Autodesk Inventor part; units mm, degrees
ref_plane "EbeneAuflage" through (-20, -13, 0) normal (0, 0, 1) x (1, 0, 0)
ref_plane "YZ Plane" through (0, 0, 0) normal (1, 0, 0) x (0, 1, 0)
ref_plane "XZ Plane" through (0, 0, 0) normal (0, 1, 0) x (-1, 0, 0)
ref_plane "EbeneBoden" through (-11.5031, -4.6031, 1.9) normal (0, 0, 1) x (1, 0, 0)
ref_plane "EbeneWändeEnde" through (17.7, 4.9, -6.9) normal (0, 0, -1) x (-1, 0, 0)
sketch "SkizzeBoden" plane through (-11.5031, -4.6031, 1.9) normal (0, 0, 1) x (1, 0, 0)
  line L0 (-7.1969, 7.4031) -> (6.8031, 7.4031)
  line L1 (6.8031, 7.4031) -> (6.8031, -7.7969)
  line L2 (6.8031, -7.7969) -> (4.3031, -7.7969)
  line L3 (4.3031, -7.7969) -> (4.3031, -6.7969)
  line L4 (4.3031, -6.7969) -> (-7.1969, -6.7969)
  line L5 (-7.1969, -6.7969) -> (-7.1969, 7.4031)
  line L6 (31.5031, 17.6031) -> (-8.4969, 17.6031)
  line L7 (-8.4969, 17.6031) -> (-8.4969, -8.3969)
  line L8 (-8.4969, -8.3969) -> (31.5031, -8.3969)
  line L9 (31.5031, -8.3969) -> (31.5031, 17.6031)
  line L10 (-18.7369, 4.6031) -> (41.7431, 4.6031)
  line L11 (11.5031, -15.8369) -> (11.5031, 25.0431)
  line L12 (-10.0969, 19.2031) -> (33.1031, 19.2031)
  line L13 (33.1031, 19.2031) -> (33.1031, -9.9969)
  line L14 (33.1031, -9.9969) -> (-10.0969, -9.9969)
  line L15 (-10.0969, -9.9969) -> (-10.0969, 19.2031)
  point P0 (11.5031, 4.6031)
  dimension "d0" = 1.6
extrude "Boden" add sketch "SkizzeBoden" along normal blind 1.5
sketch "SkizzeWände" plane through (-11.5031, -4.6031, 1.9) normal (0, 0, -1) x (-1, 0, 0)
  line L0 (10.0969, 19.2031) -> (-33.1031, 19.2031)
  line L1 (-33.1031, 19.2031) -> (-33.1031, -9.9969)
  line L2 (-33.1031, -9.9969) -> (10.0969, -9.9969)
  line L3 (10.0969, -9.9969) -> (10.0969, 19.2031)
  line L4 (-31.6031, 17.7031) -> (8.5969, 17.7031)
  line L5 (8.5969, 17.7031) -> (8.5969, -8.4969)
  line L6 (8.5969, -8.4969) -> (-31.6031, -8.4969)
  line L7 (-31.6031, -8.4969) -> (-31.6031, 17.7031)
  point P0 (-11.5031, 4.6031)
  dimension "d3" = 1.5
extrude "Wände" add sketch "SkizzeWände" along normal up to surface (8.8 mm away)
sketch "SkizzeAuflage" plane through (-11.5031, -4.6031, 1.9) normal (0, 0, -1) x (-1, 0, 0)
  line L0 (8.5969, -8.4969) -> (8.5969, 17.7031)
  line L1 (-31.6031, -8.4969) -> (8.5969, -8.4969)
  line L2 (-31.6031, 17.7031) -> (-31.6031, -8.4969)
  line L3 (8.5969, 17.7031) -> (-31.6031, 17.7031)
  line L4 (10.0969, 19.2031) -> (10.0969, -9.9969)
  line L5 (-33.1031, 19.2031) -> (10.0969, 19.2031)
  line L6 (-33.1031, -9.9969) -> (-33.1031, 19.2031)
  line L7 (10.0969, -9.9969) -> (-33.1031, -9.9969)
  line L8 (-26.6031, 3.5031) -> (-25.1031, 3.5031)
  line L9 (-25.1031, 3.5031) -> (-25.1031, -6.4969)
  line L10 (-25.1031, -6.4969) -> (-26.6031, -6.4969)
  line L11 (-26.6031, -6.4969) -> (-26.6031, 3.5031)
  line L12 (-17.1031, 3.5031) -> (-15.6031, 3.5031)
  line L13 (-15.6031, 3.5031) -> (-15.6031, -6.4969)
  line L14 (-15.6031, -6.4969) -> (-17.1031, -6.4969)
  line L15 (-17.1031, -6.4969) -> (-17.1031, 3.5031)
  line L16 (6.5969, 13.7031) -> (-13.4031, 13.7031)
  line L17 (-13.4031, 13.7031) -> (-13.4031, 12.2031)
  line L18 (-13.4031, 12.2031) -> (6.5969, 12.2031)
  line L19 (6.5969, 12.2031) -> (6.5969, 13.7031)
  point P0 (-11.5031, 4.6031)
  dimension "d6" = 5
  dimension "d7" = 1.5
  dimension "d8" = 8
  dimension "d9" = 2
  dimension "d10" = 10
  dimension "d11" = 20
  dimension "d12" = 1.5
  dimension "d13" = 4
  dimension "d14" = 2
ref_plane "EbeneAuflage" through (-20, -13, 0) normal (0, 0, 1) x (1, 0, 0)
extrude "Auflage" add sketch "SkizzeAuflage" along normal up to surface (1.9 mm away) contours L8 L9 L10 L11 | L12 L13 L14 L15 | L19 L18 L17 L16
sketch "SkizzeSD" plane through (-21.6, -14.6, 3.4) normal (0, -1, 0) x (1, 0, 0)
  line L0 (43.2, 0) -> (43.2, -10.3)
  line L1 (3.1, -2.6) -> (14.2, -2.6)
  line L2 (14.2, -2.6) -> (14.2, -1.6)
  line L3 (14.2, -1.6) -> (3.1, -1.6)
  line L4 (3.1, -1.6) -> (3.1, -2.6)
  line L5 (41.7, -1.5) -> (1.5, -1.5)
  line L6 (14.5, -1.5) -> (2.8, -1.5)
  line L7 (2.8, -1.5) -> (2.8, -2.9)
  line L8 (2.8, -2.9) -> (14.5, -2.9)
  line L9 (14.5, -2.9) -> (14.5, -1.5)
  line L10 (8.65, -4) -> (8.65, -0.8838) construction
  point P0 (21.6, -3.4)
  point P1 (8.65, -2.6)
  dimension "d17" = 0.3
  dimension "d18" = 0.3
extrude "SD" cut sketch "SkizzeSD" against normal up to surface (1.5 mm away) contours L4 L3 L2 L1 | L9 L8 L7 L5
sketch "Skizze7" plane through (-21.6, -14.6, 3.4) normal (0, -1, 0) x (1, 0, 0)
  line L0 (14.5, -1.5) -> (14.5, -2.9)
  line L1 (14.5, -2.9) -> (2.8, -2.9)
  line L2 (0, 0) -> (43.2, 0)
  line L3 (15.5, -3.9) -> (1.8, -3.9)
  line L4 (1.8, -3.9) -> (1.8, 0)
  line L5 (1.8, 0) -> (15.5, 0)
  line L6 (15.5, 0) -> (15.5, -3.9)
  line L7 (8.65, -3.6567) -> (8.65, -1) construction
  point P0 (21.6, -3.4)
  point P1 (8.65, -2.9)
  dimension "d21" = 1
  dimension "d22" = 1
extrude "SDHilfe" cut sketch "Skizze7" against normal blind 0.8
sketch "SkizzeLED" plane through (-21.6, -14.6, -6.9) normal (0, -1, 0) x (1, 0, 0)
  line L0 (16.6, 5.2) -> (17.6, 5.2)
  line L1 (16.6, 5.2) -> (16.6, 4.1)
  line L2 (17.6, 4.1) -> (16.6, 4.1)
  line L3 (17.6, 5.2) -> (17.6, 4.1)
  line L4 (15.1, 5.2) -> (16.1, 5.2)
  line L5 (15.1, 5.2) -> (15.1, 4.1)
  line L6 (16.1, 4.1) -> (15.1, 4.1)
  line L7 (16.1, 5.2) -> (16.1, 4.1)
  line L8 (13.6, 5.2) -> (14.6, 5.2)
  line L9 (13.6, 5.2) -> (13.6, 4.1)
  line L10 (14.6, 4.1) -> (13.6, 4.1)
  line L11 (14.6, 5.2) -> (14.6, 4.1)
  line L12 (15.6, 3.5363) -> (15.6, 5.4531) construction
  line L13 (17.7, 4.1) -> (13.5, 4.1)
  line L14 (13.5, 4.1) -> (13.5, 5.2)
  line L15 (13.5, 5.2) -> (17.7, 5.2)
  line L16 (17.7, 5.2) -> (17.7, 4.1)
  line L17 (41.6, 5.2) -> (1.6, 5.2)
  point P0 (21.6, 6.9)
  point P1 (15.6, 4.1)
  dimension "d25" = 0.1
extrude "LED" cut sketch "SkizzeLED" against normal up to surface (1.5 mm away)
fillet "RundungLED" radius 0.3 4 edges at (-8.1, -13.85, -2.8) (-3.9, -13.85, -2.8) (-8.1, -13.85, -1.7) (-3.9, -13.85, -1.7)
sketch "SkizzeUSB" plane through (-21.6, 14.6, 3.4) normal (0, 1, 0) x (1, 0, 0)
  line L0 (43.2, 10.3) -> (0, 10.3)
  ellipse E0 centre (28.273, 7.641) end of major axis (28.5965, 8.1263) minor radius 0.5 (28.8, 7.72) -> (28.3475, 8.2) ccw
  line L1 (28.3475, 8.2) -> (21.3525, 8.2)
  ellipse E1 centre (21.427, 7.641) end of major axis (21.1035, 8.1263) minor radius 0.5 (21.3525, 8.2) -> (20.9, 7.72) ccw
  line L2 (20.9, 7.72) -> (20.9, 6.4602)
  line L3 (22.4652, 4.8) -> (20.9, 6.4602)
  line L4 (22.4652, 4.8) -> (27.2348, 4.8)
  line L5 (28.8, 6.4602) -> (27.2348, 4.8)
  line L6 (28.8, 6.4602) -> (28.8, 7.72)
  ellipse E2 centre (28.273, 7.641) end of major axis (28.5965, 8.1263) minor radius 0.5 (28.8, 7.72) -> (28.3475, 8.2) ccw
  line L7 (28.3475, 8.2) -> (21.3525, 8.2)
  ellipse E3 centre (21.427, 7.641) end of major axis (21.1035, 8.1263) minor radius 0.5 (21.3525, 8.2) -> (20.9, 7.72) ccw
  line L8 (20.9, 7.72) -> (20.9, 6.4602)
  line L9 (22.4652, 4.8) -> (20.9, 6.4602)
  line L10 (22.4652, 4.8) -> (27.2348, 4.8)
  line L11 (28.8, 6.4602) -> (27.2348, 4.8)
  line L12 (28.8, 6.4602) -> (28.8, 7.72)
  line L13 (20.6, 10.3) -> (29.1, 10.3)
  line L14 (29.1, 10.3) -> (29.1, 4.5)
  line L15 (29.1, 4.5) -> (20.6, 4.5)
  line L16 (20.6, 4.5) -> (20.6, 10.3)
  line L17 (24.85, 8.6856) -> (24.85, 4.4469) construction
  point P0 (21.6, 3.4)
  point P1 (24.85, 8.2)
  dimension "d29" = 0.3
  dimension "d30" = 0.3
extrude "USB" cut sketch "SkizzeUSB" against normal up to surface (1.5 mm away) contours L14 L15 L16 L0 | L6 L5 L4 L3 L2 E1 L1 E0
chamfer "FaseUSB" distance 1.5 angle 45 2 edges at (7.5, 13.85, -1.1) (-1, 13.85, -1.1)
sketch "Skizze10" plane through (-21.6, -14.6, 3.4) normal (-1, 0, 0) x (0, 0, 1)
  line L0 (-10.3, 29.2) -> (-10.3, 0)
  line L1 (-5.1, 27) -> (-5.1, 12)
  line L2 (-5.1, 27) -> (-8.8, 27)
  line L3 (-8.8, 12) -> (-8.8, 27)
  line L4 (-5.1, 12) -> (-8.8, 12)
  line L5 (-5.1, 11.2) -> (-5.1, 2.2)
  line L6 (-5.1, 11.2) -> (-8.8, 11.2)
  line L7 (-8.8, 2.2) -> (-8.8, 11.2)
  line L8 (-5.1, 2.2) -> (-8.8, 2.2)
  line L9 (-4.8, 1.9) -> (-10.3, 1.9)
  line L10 (-10.3, 1.9) -> (-10.3, 27.3)
  line L11 (-10.3, 27.3) -> (-4.8, 27.3)
  line L12 (-4.8, 27.3) -> (-4.8, 1.9)
  line L13 (0, 29.2) -> (0, 0)
  line L14 (-10.3, 29.2) -> (0, 29.2)
  line L15 (3, 14.6) -> (-13.529, 14.6) construction
  line L16 (-8.4, 2.6) -> (-8.4, 10.8)
  line L17 (-8.4, 10.8) -> (-5.5, 10.8)
  line L18 (-5.5, 10.8) -> (-5.5, 2.6)
  line L19 (-5.5, 2.6) -> (-8.4, 2.6)
  line L20 (-8.4, 12.4) -> (-8.4, 26.6)
  line L21 (-8.4, 26.6) -> (-5.5, 26.6)
  line L22 (-5.5, 26.6) -> (-5.5, 12.4)
  line L23 (-5.5, 12.4) -> (-8.4, 12.4)
  point P0 (-3.4, 14.6)
  point P1 (0, 14.6)
  dimension "d36" = 0.3
  dimension "d38" = 0.3
extrude "JSTFC" cut sketch "Skizze10" against normal up to surface (1.5 mm away) contours L11 L12 L9 L0 | L1 L4 L3 L2 | L5 L8 L7 L6 | L16 L17 L18 L19 | L20 L21 L22 L23
sketch "Skizze11" plane through (21.6, -14.6, 3.4) normal (1, 0, 0) x (0, 0, -1)
  line L0 (10.3, 0) -> (10.3, 29.2)
  line L1 (13.0125, 14.6) -> (-3.6442, 14.6) construction
  line L2 (5.1, 15) -> (5.1, 24)
  line L3 (5.1, 15) -> (8.8, 15)
  line L4 (8.8, 24) -> (8.8, 15)
  line L5 (5.1, 24) -> (8.8, 24)
  line L6 (5.1, 5.2) -> (5.1, 14.2)
  line L7 (5.1, 5.2) -> (8.8, 5.2)
  line L8 (8.8, 14.2) -> (8.8, 5.2)
  line L9 (5.1, 14.2) -> (8.8, 14.2)
  line L10 (10.3, 24.3) -> (4.8, 24.3)
  line L11 (4.8, 24.3) -> (4.8, 4.9)
  line L12 (4.8, 4.9) -> (10.3, 4.9)
  line L13 (10.3, 4.9) -> (10.3, 24.3)
  line L14 (5.5, 13.8) -> (8.4, 13.8)
  line L15 (8.4, 13.8) -> (8.4, 5.6)
  line L16 (8.4, 5.6) -> (5.5, 5.6)
  line L17 (5.5, 5.6) -> (5.5, 13.8)
  line L18 (8.4, 23.6) -> (8.4, 15.4)
  line L19 (8.4, 15.4) -> (5.5, 15.4)
  line L20 (5.5, 15.4) -> (5.5, 23.6)
  line L21 (5.5, 23.6) -> (8.4, 23.6)
  point P0 (3.4, 14.6)
  point P1 (10.3, 14.6)
  dimension "d41" = 0.3
  dimension "d42" = 0.3
extrude "JSTOSD" cut sketch "Skizze11" against normal up to surface (1.5 mm away) contours L12 L11 L10 L0 | L2 L5 L4 L3 | L6 L9 L8 L7 | L14 L15 L16 L17 | L18 L19 L20 L21
sketch "Skizze12" plane through (21.6, -14.6, -6.9) normal (0, 0, -1) x (-1, 0, 0)
  line L0 (0, 0) -> (0, 4.9)
  line L1 (43.2, 0) -> (0, 0)
  line L2 (21.6, -5.84) -> (21.6, 35.04)
  line L3 (51.84, 14.6) -> (-8.64, 14.6)
  line L4 (0.8, 28.4) -> (42.4, 28.4)
  line L5 (42.4, 28.4) -> (42.4, 0.8)
  line L6 (42.4, 0.8) -> (0.8, 0.8)
  line L7 (0.8, 0.8) -> (0.8, 28.4)
  point P0 (21.6, 14.6)
  dimension "d45" = 0.8
  dimension "d46" = 0.8
extrude "Lippe" cut sketch "Skizze12" against normal blind 0.6
sketch "SkizzeSchnapper" plane through (-21.6, -14.6, -6.9) normal (0, -1, 0) x (1, 0, 0)
  line L0 (36.2, 5.2) -> (41.6, 5.2)
  line L1 (36.2, 5.2) -> (36.2, 1.5)
  line L2 (42.4, 1.5) -> (36.2, 1.5)
  line L3 (42.4, 5.2) -> (42.4, 1.5)
  line L4 (41.6, 5.2) -> (42.4, 5.2)
  line L5 (0.8, 5.2) -> (1.6, 5.2)
  line L6 (0.8, 5.2) -> (0.8, 1.5)
  line L7 (7, 1.5) -> (0.8, 1.5)
  line L8 (7, 5.2) -> (7, 1.5)
  line L9 (1.6, 5.2) -> (7, 5.2)
  ellipse E0 centre (28.273, 2.659) end of major axis (28.5965, 2.1737) minor radius 0.5 (28.3475, 2.1) -> (28.8, 2.58) ccw
  line L10 (28.3475, 2.1) -> (21.3525, 2.1)
  ellipse E1 centre (21.427, 2.659) end of major axis (21.1035, 2.1737) minor radius 0.5 (20.9, 2.58) -> (21.3525, 2.1) ccw
  line L11 (20.9, 2.58) -> (20.9, 3.8398)
  line L12 (22.4652, 5.5) -> (20.9, 3.8398)
  line L13 (22.4652, 5.5) -> (27.2348, 5.5)
  line L14 (28.8, 3.8398) -> (27.2348, 5.5)
  line L15 (28.8, 3.8398) -> (28.8, 2.58)
  line L16 (35, 2.4) -> (30.5, 2.4)
  line L17 (30.5, 2.4) -> (30.5, 4)
  line L18 (30.5, 4) -> (35, 4)
  line L19 (35, 4) -> (35, 2.4)
  line L20 (21.6, -2.06) -> (21.6, 12.36)
  line L21 (1.5, 0.6) -> (0.8, 0.6)
  line L22 (41.7, 0.6) -> (1.5, 0.6)
  line L23 (42.4, 0.6) -> (41.7, 0.6)
  line L24 (0.8, 0.6) -> (42.4, 0.6)
  line L25 (41.6, 5.2) -> (1.6, 5.2)
  line L26 (8.2, 2.4) -> (12.7, 2.4)
  line L27 (12.7, 2.4) -> (12.7, 4)
  line L28 (12.7, 4) -> (8.2, 4)
  line L29 (8.2, 4) -> (8.2, 2.4)
  point P0 (21.6, 6.9)
  dimension "d49" = 4.5
  dimension "d50" = 1.8
  dimension "d51" = 1.2
  dimension "d52" = 1.6
  dimension "d53" = 1.2
extrude "Schnapper" cut sketch "SkizzeSchnapper" against normal up to surface (29.2 mm away) contours L16 L17 L18 L19 | L29 L28 L27 L26
sketch "SkizzeAufkleber" plane through (-11.5031, -4.6031, 3.4) normal (0, 0, 1) x (1, 0, 0)
  line L0 (33.1031, 19.2031) -> (-10.0969, 19.2031)
  line L1 (-10.0969, 19.2031) -> (-10.0969, -9.9969)
  line L2 (11.5031, -15.8369) -> (11.5031, 25.0431)
  line L3 (-18.7369, 4.6031) -> (41.7431, 4.6031)
  line L4 (-8.0969, 17.2031) -> (31.1031, 17.2031)
  line L5 (31.1031, 17.2031) -> (31.1031, -7.9969)
  line L6 (31.1031, -7.9969) -> (-8.0969, -7.9969)
  line L7 (-8.0969, -7.9969) -> (-8.0969, 17.2031)
  point P0 (11.5031, 4.6031)
  dimension "d56" = 2
  dimension "d57" = 2
extrude "Aufkleber" cut sketch "SkizzeAufkleber" against normal blind 0.3 contours L4 L5 L3 L2 | L2 L3 L7 L4 | L3 L5 L6 L2 | L2 L6 L7 L3
properties part number "Boden"
Work out the finished part from the listing and answer in its coordinate system (mm). A direction names the side the tool comes from. Coordinates: 2 decimals unless noted, no trailing zeros. Order: outer loops, then holes, each group sorted by start corner. A loop starts at its lowest first (then second) coordinate and runs counter-clockwise, first axis right, second up. Notation, with made-up numbers: (30, 17.25) - (35, 17.25) arc R20 ccw to (35, 42.25) - close; hole circle Ø3 at (-20.75, -37.5). An arc over 180 degrees is marked (long way). Put each result on its own line as item: value. Start each with the question number.
1) For a pull along X with two mould halves and no side action, classify faces 1 (the flat face through (-0.3, 14.6, -1.68)), 2 (the flat face through (-11, 14, -2.9)) as released by +X, released by -X, zero draft, split by the parting line, or undercut.
2) Find section A-A (x = -16.5). Give the vertices of the cut face in (y, z), plus the area to 4 significant figures.
3) Find section D-D (y = -12). Give the vertices of the cut face in (x, z), plus the area to 3 significant figures.
4) Find section B-B (z = 1.25). Give the vertices of the cut face in (x, y).
5) For faces 3 (the flat face through (-13, -13.8, 2.3)), 4 (the flat face through (11, 14, -4.5)), 5 (the flat face through (21, -9.7, -4)), 6 (the flat face through (-21, -12.7, -4)), 7 (the flat face through (-8, 9.1, 1)), determine the directions among +Z, -Z, +X, -X, +Y, -Y from which every point of the face is accessible in a straight line to the end or side of a thin tool.
6) Find the intervals of material crossed by line 1 (Y direction, x = -1.5, z = 1.5); line 2 (X direction, y = -2.75, z = 3.25); line 3 (X direction, y = 2.25, z = 0.25), in increasing order. Write a range as from..to.
7) Flat-ended cylindrical pins translate along their axes: pin 1 (5 mm diameter, centred on x = 3, y = -10, fed in from +Z); pin 2 (0.6 mm diameter, centred on x = -10.5, z = 1, fed in from -Y); pin 3 (3 mm diameter, centred on y = -10, z = -5.5, fed in from -X). Find the tip coordinate at first contact, or state that the pin passes through.
8) Find section C-C (x = 11.5). Give the vertices of the cut face in (y, z).
Results list:
1. face 1: zero draft
1. face 2: undercut
2. outline: (-14.6, -6.9) - (-13.8, -6.9) - (-13.8, -6.3) - (-13.1, -6.3) - (-13.1, 0.5) - (-13.8, 0.5) - (-13.8, -0.5) - (-14.6, -0.5) - close; (-13.8, 1.9) - (7.6, 1.9) - (7.6, 0) - (9.1, 0) - (9.1, 1.9) - (13.1, 1.9) - (13.1, -6.3) - (13.8, -6.3) - (13.8, -6.9) - (14.6, -6.9) - (14.6, 3.4) - (12.6, 3.4) - (12.6, 3.1) - (-12.6, 3.1) - (-12.6, 3.4) - (-13.8, 3.4) - close
2. area: 60.55 mm^2
3. outline: (-21.6, -1.4) - (-20.1, -1.4) - (-20.1, 1.9) - (20.1, 1.9) - (20.1, -6.3) - (20.8, -6.3) - (20.8, -6.9) - (21.6, -6.9) - (21.6, 3.4) - (19.6, 3.4) - (19.6, 3.1) - (-19.6, 3.1) - (-19.6, 3.4) - (-21.6, 3.4) - close
3. area: 70.8 mm^2
4. outline: (-21.6, -14.6) - (-19.8, -14.6) - (-19.8, -13.8) - (-18.8, -13.8) - (-18.8, -13.1) - (-20.1, -13.1) - (-20.1, 13.1) - (20.1, 13.1) - (20.1, -13.1) - (-7.1, -13.1) - (-7.1, -13.8) - (-6.1, -13.8) - (-6.1, -14.6) - (21.6, -14.6) - (21.6, 14.6) - (-21.6, 14.6) - close; (-18.1, 7.6) - (1.9, 7.6) - (1.9, 9.1) - (-18.1, 9.1) - close; (4.1, -11.1) - (5.6, -11.1) - (5.6, -1.1) - (4.1, -1.1) - close; (13.6, -11.1) - (15.1, -11.1) - (15.1, -1.1) - (13.6, -1.1) - close
5. face 3: +Z, -Y
5. face 4: +Y, -Y
5. face 5: -Z, +X, -X
5. face 6: -Z, -X
5. face 7: -Z
6. line 1: y = -14.6..-13.1, 7.6..9.1, 13.1..14.6
6. line 2: x = -21.6..-19.6, 19.6..21.6
6. line 3: x = -21.6..-20.1, 20.1..21.6
7. pin 1: stops at z = 3.1
7. pin 2: stops at y = 7.6
7. pin 3: stops at x = 20.1
8. outline: (-14.6, -6.9) - (-13.8, -6.9) - (-13.8, -6.3) - (-13.1, -6.3) - (-13.1, -4.5) - (-14.6, -4.5) - close; (-14.6, -2.9) - (-13.1, -2.9) - (-13.1, 1.9) - (13.1, 1.9) - (13.1, -2.9) - (14.6, -2.9) - (14.6, 3.4) - (12.6, 3.4) - (12.6, 3.1) - (-12.6, 3.1) - (-12.6, 3.4) - (-14.6, 3.4) - close; (13.1, -6.3) - (13.8, -6.3) - (13.8, -6.9) - (14.6, -6.9) - (14.6, -4.5) - (13.1, -4.5) - close
